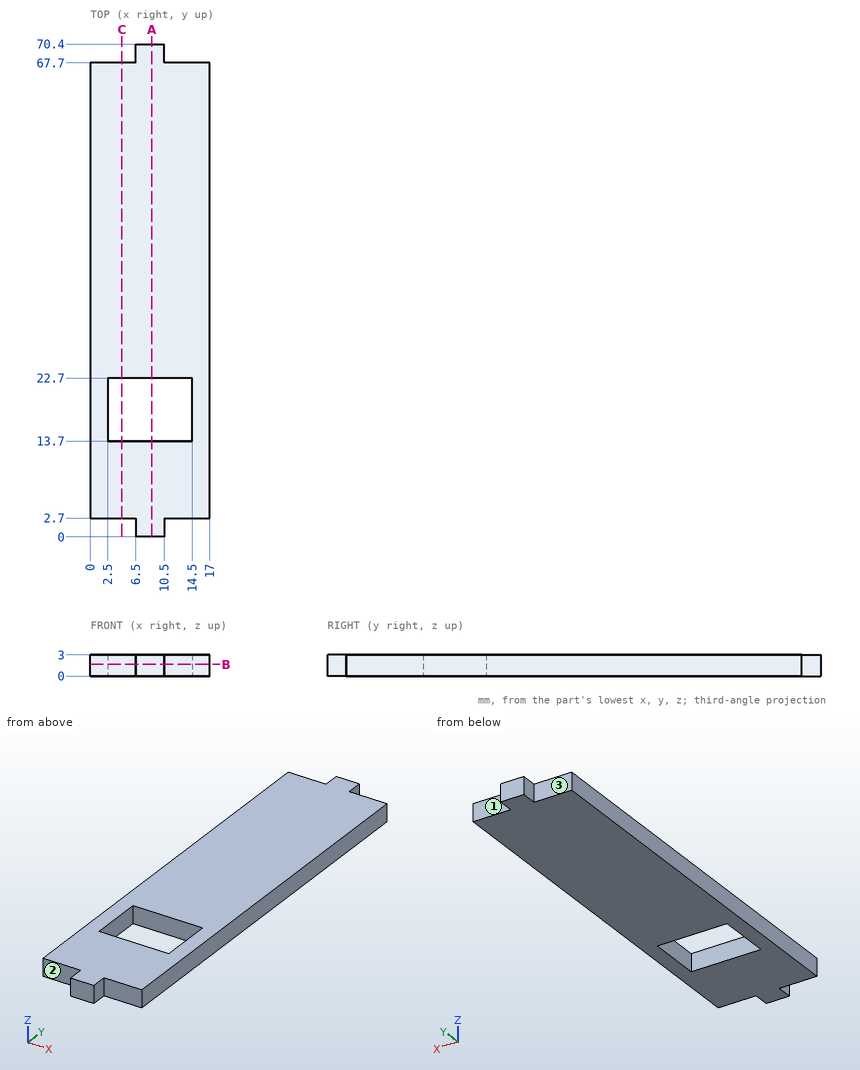
The figure shows three views and two pictorial views of one solid part (mm, origin at its lowest corner). Answer the questions. A direction names the side the tool comes from. Coordinates: 2 decimals unless noted, no trailing zeros. Loops run counter-clockwise (first coordinate to the right, second up) from the corner with the lowest first, then second, coordinate; pieces in that order, holes last. Notation, with made-up numbers: (50, 41) - (63, 41) arc R17 ccw to (63, 70) - close; hole circle Ø10 at (39, 79.25). An arc over 180 degrees is marked (long way). Write item = value, one per line.
1) Which of the six approach directions +Z, -Z, +X, -X, +Y, -Y give full straight-line access (tool end or side, diameter ignored) to the marked faces 1, 2 and 3?
Responses:
face_1 = +Z, -Z, +X, +Y
face_2 = +Z, -Z, -X, -Y
face_3 = +Z, -Z, -X, +Y
2) Section C-C (x = 4.5) is taken. Determine the outline of the cut face in (y, z), plus the area to 3 significant figures.
Responses:
outline = (2.7, 0) - (13.7, 0) - (13.7, 3) - (2.7, 3) - close; (22.7, 0) - (67.7, 0) - (67.7, 3) - (22.7, 3) - close
area = 168 mm^2
3) Section B-B (z = 1.65) is taken. Determine the outline of the cut face in (x, y).
Responses:
outline = (0, 2.7) - (6.5, 2.7) - (6.5, 0) - (10.5, 0) - (10.5, 2.7) - (17, 2.7) - (17, 67.7) - (10.5, 67.7) - (10.5, 70.4) - (6.5, 70.4) - (6.5, 67.7) - (0, 67.7) - close; hole (2.5, 13.7) - (14.5, 13.7) - (14.5, 22.7) - (2.5, 22.7) - close
4) Each of these flat-tipped pins is pushed along its axis until it touches: P1, Ø0.9, axis at x = 1.5, z = 1.5, coming from the +Y side; P2, Ø5, axis at x = 5, y = 48, coming from the -Z side; P3, Ø1, axis at x = 2, z = 2, coming from the -Y side. Where does it stop, or does it pass through?
Responses:
P1 = 67.7
P2 = 0
P3 = 2.7
5) Section A-A (x = 8.75) is taken. Determine the outline of the cut face in (y, z).
Responses:
outline = (0, 0) - (13.7, 0) - (13.7, 3) - (0, 3) - close; (22.7, 0) - (70.4, 0) - (70.4, 3) - (22.7, 3) - close
6) Find the intervals of material crossed by line 1 along Y through (x, z) = (6.25, 0.9); line 2 along Y through (x, z) = (7.5, 1.8); line 3 along X through (y, z) = (20, 1), in increasing order.
Responses:
line_1 = 2.7 to 13.7, 22.7 to 67.7
line_2 = 0 to 13.7, 22.7 to 70.4
line_3 = 0 to 2.5, 14.5 to 17
